```python
from build123d import *

# Parameters (mm, degrees)
EXTRUDE_1_DEPTH      = 257.5
EXTRUDE_1_DEPTH_BACK = 257.5
SKETCH_1_W           = 15
SKETCH_1_H           = 15
SKETCH_1_W_2         = 13
SKETCH_1_H_2         = 13
SKETCH_2_R           = 1.25
SKETCH_2_R_2         = 1.5
CUT_EXTRUDE_1_DEPTH  = 259.045538617


with BuildPart() as part:
    # 草图1 → 凸台-拉伸1 (new, two sides: drawn at the far end of the back side and taken through both)
    with BuildSketch(Plane(origin=(0, 0, 0), x_dir=(0, 0, -1), z_dir=(1, 0, 0)).offset(-EXTRUDE_1_DEPTH_BACK)):
        Rectangle(SKETCH_1_W, SKETCH_1_H)
        Rectangle(SKETCH_1_W_2, SKETCH_1_H_2, mode=Mode.SUBTRACT)
    extrude(amount=EXTRUDE_1_DEPTH + EXTRUDE_1_DEPTH_BACK)

    # 草图2 → 切除-拉伸1 (cut, through all)
    with BuildSketch(Plane(origin=(0, 0, -7.5), x_dir=(-1, 0, 0), z_dir=(0, 0, -1))):
        with Locations((-243.21681474, -4.5)):
            Circle(SKETCH_2_R)
        with Locations((-253.5, 0)):
            Circle(SKETCH_2_R_2)
        with Locations((253.5, 0)):
            Circle(SKETCH_2_R_2)
        with Locations((-239.5, 0)):
            Circle(SKETCH_2_R_2)
        with Locations((-229.5, 0)):
            Circle(SKETCH_2_R_2)
        with Locations((229.5, 0)):
            Circle(SKETCH_2_R_2)
        with Locations((239.5, 0)):
            Circle(SKETCH_2_R_2)
        with Locations((-89.5, 0)):
            Circle(SKETCH_2_R_2)
        with Locations((-79.5, 0)):
            Circle(SKETCH_2_R_2)
        with Locations((79.5, 0)):
            Circle(SKETCH_2_R_2)
        with Locations((89.5, 0)):
            Circle(SKETCH_2_R_2)
        with Locations((-224.37681474, -4.5)):
            Circle(SKETCH_2_R)
        with Locations((-205.53681474, -4.5)):
            Circle(SKETCH_2_R)
        with Locations((-186.69681474, -4.5)):
            Circle(SKETCH_2_R)
        with Locations((-167.85681474, -4.5)):
            Circle(SKETCH_2_R)
        with Locations((-149.01681474, -4.5)):
            Circle(SKETCH_2_R)
        with Locations((-130.17681474, -4.5)):
            Circle(SKETCH_2_R)
        with Locations((-111.33681474, -4.5)):
            Circle(SKETCH_2_R)
        with Locations((-92.49681474, -4.5)):
            Circle(SKETCH_2_R)
        with Locations((-73.65681474, -4.5)):
            Circle(SKETCH_2_R)
        with Locations((-54.81681474, -4.5)):
            Circle(SKETCH_2_R)
        with Locations((-35.97681474, -4.5)):
            Circle(SKETCH_2_R)
        with Locations((-17.13681474, -4.5)):
            Circle(SKETCH_2_R)
        with Locations((1.70318526, -4.5)):
            Circle(SKETCH_2_R)
        with Locations((20.54318526, -4.5)):
            Circle(SKETCH_2_R)
        with Locations((39.38318526, -4.5)):
            Circle(SKETCH_2_R)
        with Locations((58.22318526, -4.5)):
            Circle(SKETCH_2_R)
        with Locations((77.06318526, -4.5)):
            Circle(SKETCH_2_R)
        with Locations((95.90318526, -4.5)):
            Circle(SKETCH_2_R)
        with Locations((114.74318526, -4.5)):
            Circle(SKETCH_2_R)
        with Locations((133.58318526, -4.5)):
            Circle(SKETCH_2_R)
        with Locations((152.42318526, -4.5)):
            Circle(SKETCH_2_R)
        with Locations((171.26318526, -4.5)):
            Circle(SKETCH_2_R)
        with Locations((190.10318526, -4.5)):
            Circle(SKETCH_2_R)
        with Locations((208.94318526, -4.5)):
            Circle(SKETCH_2_R)
        with Locations((227.78318526, -4.5)):
            Circle(SKETCH_2_R)
        with Locations((246.62318526, -4.5)):
            Circle(SKETCH_2_R)
        with Locations((265.46318526, -4.5)):
            Circle(SKETCH_2_R)
        with Locations((284.30318526, -4.5)):
            Circle(SKETCH_2_R)
        with Locations((303.14318526, -4.5)):
            Circle(SKETCH_2_R)
    extrude(amount=-CUT_EXTRUDE_1_DEPTH, mode=Mode.SUBTRACT)


solid = part.part
```
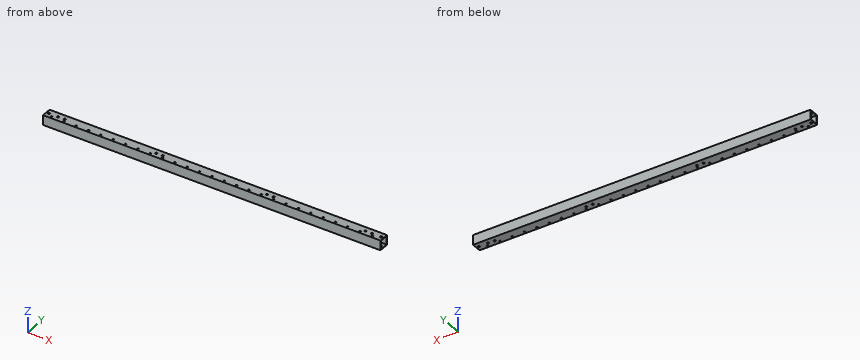
Geometry check sheet. Reference: the model listing, model coordinates, mm. Round coordinates to 2 decimals unless told otherwise and drop trailing zeros. Order: outer loops, then holes, each group sorted by start corner. A loop starts at its lowest first (then second) coordinate and runs counter-clockwise, first axis right, second up. Notation, with made-up numbers: (35.25, -26) - (44.25, -26) arc R15 cw to (44.25, -22) - close; hole circle Ø3 at (11.5, 24). An arc over 180 degrees is marked (long way). Use a Markdown table: item, result. Add a question column.
(1) Sectioned sample at B-B, the plane x = 159. Enter the section's corners in (y, z), and give its area (3 significant figures).
(2) Sectioned sample at A-A, the plane z = -3. Enter the section's corners in (x, y).
(3) Depth check by flat-ended pin: pin 1 (1.5 mm diameter, centred on x = 205.54, y = -4.5, fed in from -Z). Enter the tip coordinate at first touch or a pass-through.
(4) Material ranges on line 1 along Z through (x, y) = (100.5, 1); line 2 along Y through (x, z) = (79.5, 7.1), recorded low to high. Write a range as [from, to].
Answers below:
| question | item | result |
|---|---|---|
| 1 | outline | (-7.5, -7.5) - (7.5, -7.5) - (7.5, 7.5) - (-7.5, 7.5) - close; hole (-6.5, -6.5) - (6.5, -6.5) - (6.5, 6.5) - (-6.5, 6.5) - close |
| 1 | area | 56.0 mm² |
| 2 | outline | (-257.5, -7.5) - (257.5, -7.5) - (257.5, -6.5) - (-257.5, -6.5) - close; (-257.5, 6.5) - (257.5, 6.5) - (257.5, 7.5) - (-257.5, 7.5) - close |
| 3 | pin 1 | through |
| 4 | line 1 | [-7.5, -6.5], [6.5, 7.5] |
| 4 | line 2 | [-7.5, -1.5], [1.5, 7.5] |
